Geometry check sheet. Reference: the model listing, model coordinates, mm. A direction names the side the tool comes from. Give positions to 0.01 mm unless a question says otherwise; leave off trailing zeros. Order: outer loops, then holes, each group sorted by start corner. A loop starts at its lowest first (then second) coordinate and runs counter-clockwise, first axis right, second up. Notation, with made-up numbers: M -23,80 L 0,80 A27 ccw 0,119 Z; hole C 0.25,30.25 d9. An arc over 180 degrees is marked long. Put each result on its own line as item: value. Start each with the question number.
Q1. Section check B-B on z = 95. Record the cut outline in (x, y).
Q2. Go/stop test with flat-tipped pins: pin 1 (1.5 mm diameter, centred on x = 67.5, z = -56.5, fed in from -Y); pin 2 (6 mm diameter, centred on x = -15.5, y = 33.5, fed in from +Z); pin 3 (13 mm diameter, centred on x = -95, z = -95, fed in from +Y); pin 4 (1.5 mm diameter, centred on x = 54, z = 46.5, fed in from +Y). Record where each tip stops, or that it passes through.
Q3. Section check A-A on x = 95. Record the cut outline in (y, z).
Q4. Access from +Z, -Z, +X, -X, +Y, -Y to the whole of each face (thin tool, end or side, straight path). Record for faces 4 (the flat face through (0, 15, -97)), 5 (the flat face through (90, 27, -1)), 6 (the flat face through (-1, 27, -90)).
Q5. Section check D-D on x = 0. Record the cut outline in (y, z).
Q6. Mould release check, pull along Z, two halves, no side actions. Record for faces 1 (the flat face through (100, 7, -1)), 2 (the flat face through (1, 27, 90)), 3 (the cylindrical face through (-95.867, 7.395, -98.905)): +Z half, -Z half, draft (parallel to the pull), parting line (faces both ways), or undercut.
Q7. Material ranges on L1, parallel to Z at x = -95, y = 3.25; L2, parallel to Y at x = -33, z = -12.5, recorded low to high.
Q8. Section check C-C on z = 0. Record the cut outline in (x, y).
Autodesk Fusion 360 part; units mm, degrees
sketch "Sketch1" plane through (0, 0, 0) normal (0, 1, 0) x (1, 0, 0)
  line L0 (90, -90) -> (-90, -90)
  line L1 (-90, -90) -> (-90, 90)
  line L2 (-90, 90) -> (90, 90)
  line L3 (90, 90) -> (90, -90)
  line L4 (90, -90) -> (-90, 90) construction
  line L5 (-90, -90) -> (90, 90) construction
  line L6 (100, -100) -> (-100, -100)
  line L7 (-100, -100) -> (-100, 100)
  line L8 (-100, 100) -> (100, 100)
  line L9 (100, 100) -> (100, -100)
  line L10 (100, -100) -> (-100, 100) construction
  line L11 (-100, -100) -> (100, 100) construction
  line L12 (-100, 100) -> (-90, 90)
  line L13 (100, 100) -> (90, 90)
  line L14 (90, -90) -> (100, -100)
  line L15 (-90, -90) -> (-100, -100)
  circle A0 centre (-95, -95) radius 4
  circle A1 centre (-95, 95) radius 4
  circle A2 centre (95, 95) radius 4
  circle A3 centre (95, -95) radius 4
  dimension "d3" = 180
  dimension "d4" = 180
  dimension "d5" = 200
  dimension "d6" = 200
  dimension "d7" = 8
  dimension "d8" = 8
  dimension "d9" = 8
  dimension "d10" = 8
extrude "Extrude1" add sketch "Sketch1" along normal blind 40 contours L0 L1 L2 L3
extrude "Extrude2" add sketch "Sketch1" along normal blind 15 contours L0 L6 L14 L15 A0 A3 | L3 L9 L13 L14 A2 A3 | L1 L7 L12 L15 A0 A1 | L2 L8 L12 L13 A1 A2
sketch "Sketch2" plane through (0, 40, 0) normal (0, 1, 0) x (-1, 0, 0)
  line L0 (-90, -90) -> (90, -90)
  line L1 (90, -90) -> (90, 90)
  line L2 (90, 90) -> (-90, 90)
  line L3 (-90, 90) -> (-90, -90)
  circle A0 centre (0, 0) radius 87.5
  circle A1 centre (0, 0) radius 12.5
  dimension "d15" = 175
  dimension "d16" = 25
extrude "Extrude3" add sketch "Sketch2" along normal blind 30 contours A1
extrude "Extrude4" add sketch "Sketch2" along normal blind 10 contours A0
fillet "Fillet1" radius 2.5 1 edges at (81.5786, 50, -31.6414)
sketch "Sketch3" plane through (0, 50, 0) normal (0, 1, 0) x (-1, 0, 0)
  circle A0 centre (0, 0) radius 12.5
  circle A1 centre (0, 0) radius 85
Results found:
1. outline: M -100,0 L -99,0 L -99,15 L -100,15 Z; M -91,0 L 91,0 L 91,15 L -91,15 Z; M 99,0 L 100,0 L 100,15 L 99,15 Z
2. pin 1: stops at y = 0
2. pin 2: stops at z = 90
2. pin 3: stops at y = 15
2. pin 4: stops at y = 50
3. outline: M 0,-100 L 15,-100 L 15,-99 L 0,-99 Z; M 0,-91 L 15,-91 L 15,91 L 0,91 Z; M 0,99 L 15,99 L 15,100 L 0,100 Z
4. face 4: +Y
4. face 5: +Z, -Z, +X, +Y
4. face 6: -Z, +X, -X, +Y
5. outline: M 0,-100 L 15,-100 L 15,-90 L 40,-90 L 40,-87.5 L 47.5,-87.5 A2.5 ccw 50,-85 L 50,-12.5 L 70,-12.5 L 70,12.5 L 50,12.5 L 50,85 A2.5 ccw 47.5,87.5 L 40,87.5 L 40,90 L 15,90 L 15,100 L 0,100 Z
6. face 1: draft
6. face 2: +Z half
6. face 3: undercut
7. L1: z = -100 to -99, -91 to 91, 99 to 100
7. L2: y = 0 to 50
8. outline: M -100,0 L 100,0 L 100,15 L 90,15 L 90,40 L 87.5,40 L 87.5,47.5 A2.5 ccw 85,50 L 12.5,50 L 12.5,70 L -12.5,70 L -12.5,50 L -85,50 A2.5 ccw -87.5,47.5 L -87.5,40 L -90,40 L -90,15 L -100,15 Z
